Print and shaded views of the part. All mm, measured from the part's lowest x, y and z. A direction names the side the tool comes from. Give positions to 0.01 mm unless a question says otherwise; leave off trailing zeros. Write each loop counter-clockwise with the first axis right and the second up, starting at its lowest first coordinate (ties: lowest second). Pieces come first, ordered by that corner, then holes. Notation, with made-up numbers: (-13, 0) -> (-6, 0) arc R16 ccw to (-6, 5) -> close; hole circle Ø6 at (62, 78). An arc over 180 degrees is marked (long way). Put each result on its own line as item: value.
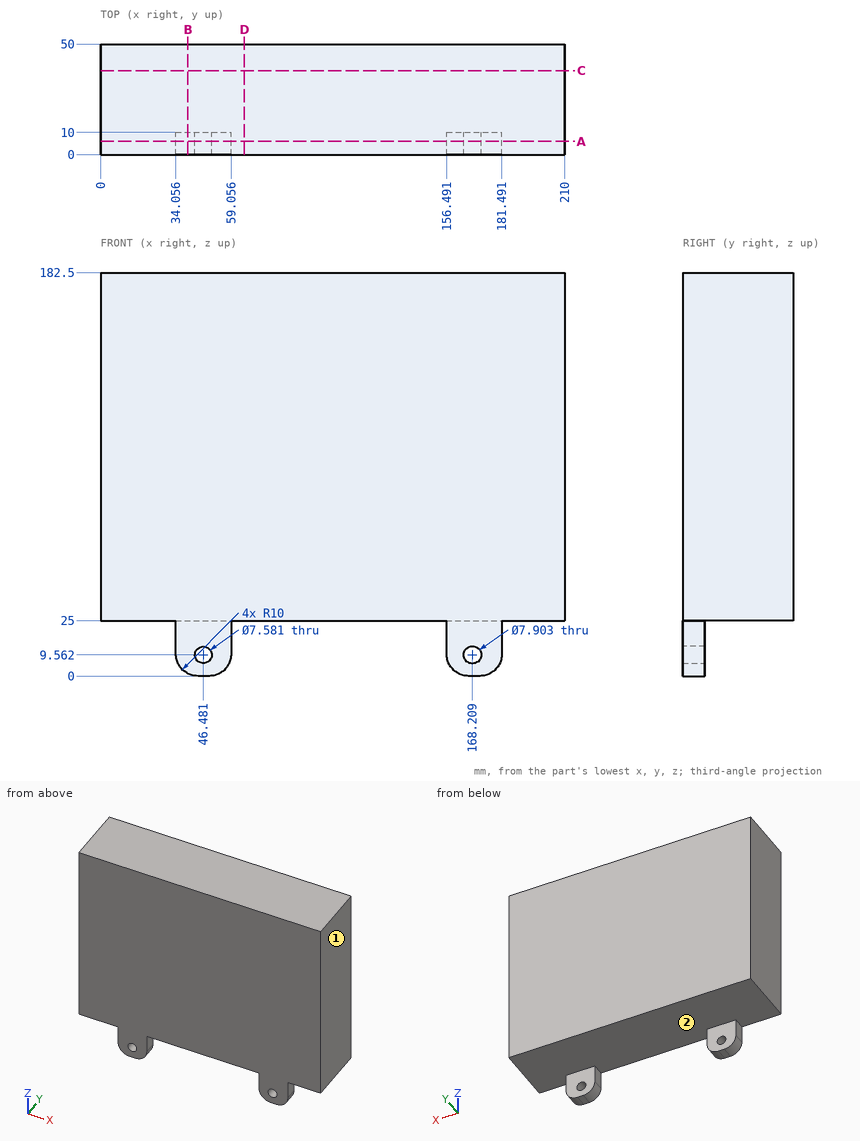
1) Slice it at D-D (x = 65). Write the cut outline in (y, z).
Filled sheet:
outline: (0, 25) -> (50, 25) -> (50, 182.5) -> (0, 182.5) -> close
2) Slice it at B-B (x = 39.5). Write the cut outline in (y, z).
Filled sheet:
outline: (0, 1.1) -> (10, 1.1) -> (10, 25) -> (50, 25) -> (50, 182.5) -> (0, 182.5) -> close
3) Tool access for the marked faces 1 and 2: list every direction of +Z, -Z, +X, -X, +Y, -Y with a clear straight run to the whole face (end or side of a thin tool).
Filled sheet:
face 1: +Z, -Z, +X, +Y, -Y
face 2: -Z, +Y
4) Wall check: L1, parallel to Y at x = 37.5, z = 20; L2, parallel to Z at x = 167, y = 21. Give the ranges that are in metal, low to high.
Filled sheet:
L1: 0 to 10
L2: 25 to 182.5
5) Pin check, flat tips, straight feed: pin 1 (11 mm diameter, centred on y = 4.5, z = 17, fed in from +X); pin 2 (4.5 mm diameter, centred on x = 46.48, z = 9.56, fed in from +Y) (1 decimal); pin 3 (8 mm diameter, centred on y = 2.5, z = 20.5, fed in from -X); pin 4 (15 mm diameter, centred on x = 62, y = 33.5, fed in from -Z). Stop position of each tip, or through.
Filled sheet:
pin 1: x = 181.49
pin 2: through
pin 3: x = 34.06
pin 4: z = 25
6) Slice it at A-A (y = 6). Write the cut outline in (x, z).
Filled sheet:
outline: (0, 25) -> (34.06, 25) -> (34.06, 10) arc R10 ccw to (44.06, 0) -> (49.06, 0) arc R10 ccw to (59.06, 10) -> (59.06, 25) -> (156.49, 25) -> (156.49, 10) arc R10 ccw to (166.49, 0) -> (171.49, 0) arc R10 ccw to (181.49, 10) -> (181.49, 25) -> (210, 25) -> (210, 182.5) -> (0, 182.5) -> close; hole circle Ø7.58 at (46.48, 9.56); hole circle Ø7.9 at (168.21, 9.56)
7) Slice it at C-C (y = 38). Write the cut outline in (x, z).
Filled sheet:
outline: (0, 25) -> (210, 25) -> (210, 182.5) -> (0, 182.5) -> close
